Geometry check sheet. Reference: the model listing, model coordinates, mm. A direction names the side the tool comes from. Round coordinates to 2 decimals unless told otherwise and drop trailing zeros. Loops run counter-clockwise (first coordinate to the right, second up) from the corner with the lowest first, then second, coordinate; pieces in that order, holes last. Notation, with made-up numbers: (-10, 75) -> (10, 75) arc R10 ccw to (10, 81) -> close; hole circle Ø6 at (46.25, -24.75). An arc over 180 degrees is marked (long way). Use a Markdown table: item, result. Add a question column.
Q1. Gauge pin test, flat ends, axial feed: P1, Ø7.5, axis at y = -53, z = -84, coming from the +X side; P2, Ø2, axis at y = -48, z = -100.5, coming from the -X side; P3, Ø13, axis at x = 10.5, y = -29, coming from the +Z side. Record the tip position at first contact, or that the pin passes through.
Q2. Sectioned sample at C-C, the plane y = -38. Enter the section's corners in (x, z).
Q3. Sectioned sample at B-B, the plane x = 0. Enter the section's corners in (y, z), then the cut area to 3 significant figures.
Q4. Release check for a two-part mould opening along Z. For faces 6 (the face through (-1, -47, -8)), 7 (the face through (-1, -34, -130)), 8 (the face through (0.1, -26.5, -82)), 9 (the face through (0, -57, -68)) record: released by +Z, released by -Z, zero draft, split by the parting line, or undercut.
Q5. Material ranges on L1, parallel to X at y = -45, z = -81; L2, parallel to Y at x = -32, z = -87; L3, parallel to Z at x = 13, y = -33, recorded low to high.
Q6. Set-up check for faces 1 (the face through (22, -20.25, -70)), 2 (the face through (-0.5, -25.2, -49)), 3 (the face through (0, -30, -24)), 4 (the face through (33, -42, -70)), 5 (the face through (-32, -42, -70)): record each of +Z, -Z, +X, -X, +Y, -Y from which the full face is reachable in a straight line by a thin tool's end or side.
Q7. Sectioned sample at A-A, the plane z = -29.5. Enter the section's corners in (x, y), then the cut area to 3 significant figures.
Q8. Sectioned sample at D-D, the plane y = -49. Enter the section's corners in (x, z).
```python
from build123d import *

# Parameters (mm, degrees)
BOSS_EXTRUDE1_DEPTH     = 8
SKETCH3_R               = 13.75
CUT_EXTRUDE1_DEPTH      = 8
SKETCH4_W               = 80
SKETCH4_H               = 37
BOSS_EXTRUDE2_DEPTH     = 122
SKETCH5_R               = 26.5
CUT_EXTRUDE2_DEPTH      = 16
SKETCH6_R               = 6.5
CUT_EXTRUDE3_DEPTH      = 122
BOSS_EXTRUDE3_START     = 16
BOSS_EXTRUDE3_DEPTH     = 25
BOSS_EXTRUDE4_START     = 108
BOSS_EXTRUDE4_DEPTH     = 14
SKETCH10_W              = 150
SKETCH10_H              = 175
CUT_EXTRUDE4_DEPTH      = 8
CUT_EXTRUDE5_DEPTH      = 141.474196919
CUT_EXTRUDE5_DEPTH_BACK = 141.474196919
SKETCH12_W              = 80
SKETCH12_H              = 0.25
SKETCH13_W              = 15
SKETCH13_H              = 15
CUT_EXTRUDE6_DEPTH      = 122


with BuildPart() as part:
    # Sketch2 → Boss-Extrude1 (new body)
    with BuildSketch(Plane.XY):
        with BuildLine():
            Line((-35, 60), (-35, 50))
            ThreePointArc((-35, 50), (-37.196699141, 44.696699141), (-42.5, 42.5))
            Line((-42.5, 42.5), (-52.5, 42.5))
            ThreePointArc((-52.5, 42.5), (-57.803300859, 40.303300859), (-60, 35))
            Line((-60, 35), (-60, -60))
            ThreePointArc((-60, -60), (-57.803300859, -65.303300859), (-52.5, -67.5))
            Line((-52.5, -67.5), (52.5, -67.5))
            ThreePointArc((52.5, -67.5), (57.803300859, -65.303300859), (60, -60))
            Line((60, -60), (60, 35))
            ThreePointArc((60, 35), (57.803300859, 40.303300859), (52.5, 42.5))
            Line((52.5, 42.5), (42.5, 42.5))
            ThreePointArc((42.5, 42.5), (37.196699141, 44.696699141), (35, 50))
            Line((35, 50), (35, 60))
            ThreePointArc((35, 60), (32.803300859, 65.303300859), (27.5, 67.5))
            Line((27.5, 67.5), (-27.5, 67.5))
            ThreePointArc((-27.5, 67.5), (-32.803300859, 65.303300859), (-35, 60))
        make_face()
    extrude(amount=-BOSS_EXTRUDE1_DEPTH)

    # Sketch3 → Cut-Extrude1 (cut)
    with BuildSketch(Plane.XY):
        with Locations((0, -20)):
            Circle(SKETCH3_R)
    extrude(amount=-CUT_EXTRUDE1_DEPTH, mode=Mode.SUBTRACT)

    # Sketch4 → Boss-Extrude2 (add)
    with BuildSketch(Plane(origin=(0, 0, -8), x_dir=(-1, 0, 0), z_dir=(0, 0, -1))):
        with Locations((0, -38.5)):
            Rectangle(SKETCH4_W, SKETCH4_H)
    extrude(amount=BOSS_EXTRUDE2_DEPTH)

    # Sketch5 → Cut-Extrude2 (cut)
    with BuildSketch(Plane(origin=(0, 0, -8), x_dir=(-1, 0, 0), z_dir=(0, 0, -1))):
        with Locations((0, -20)):
            Circle(SKETCH5_R)
    extrude(amount=CUT_EXTRUDE2_DEPTH, mode=Mode.SUBTRACT)

    # Sketch6 → Cut-Extrude3 (cut)
    with BuildSketch(Plane(origin=(0, 0, -8), x_dir=(-1, 0, 0), z_dir=(0, 0, -1))):
        with Locations((0, -20)):
            Circle(SKETCH6_R)
    extrude(amount=CUT_EXTRUDE3_DEPTH, mode=Mode.SUBTRACT)

    # Sketch8 → Boss-Extrude3 (add)
    with BuildSketch(Plane(origin=(0, 0, -8), x_dir=(-1, 0, 0), z_dir=(0, 0, -1)).offset(BOSS_EXTRUDE3_START)):
        with BuildLine():
            Line((-6.5, -20), (-5, -20))
            ThreePointArc((-5, -20), (0, -25), (5, -20))
            Line((5, -20), (6.5, -20))
            ThreePointArc((6.5, -20), (0, -26.5), (-6.5, -20))
        make_face()
    extrude(amount=BOSS_EXTRUDE3_DEPTH)

    # Sketch9 → Boss-Extrude4 (add)
    with BuildSketch(Plane(origin=(0, 0, -8), x_dir=(-1, 0, 0), z_dir=(0, 0, -1)).offset(BOSS_EXTRUDE4_START)):
        with BuildLine():
            Line((-6.5, -20), (-5, -20))
            ThreePointArc((-5, -20), (0, -25), (5, -20))
            Line((5, -20), (6.5, -20))
            ThreePointArc((6.5, -20), (0, -26.5), (-6.5, -20))
        make_face()
    extrude(amount=BOSS_EXTRUDE4_DEPTH)

    # Sketch10 → Cut-Extrude4 (cut)
    with BuildSketch(Plane.XY):
        Rectangle(SKETCH10_W, SKETCH10_H)
    extrude(amount=-CUT_EXTRUDE4_DEPTH, mode=Mode.SUBTRACT)

    # Sketch12 → Cut-Extrude5 (cut, two sides: drawn at the far end of the back side and taken through both)
    with BuildSketch(Plane.XY.offset(-8).offset(-CUT_EXTRUDE5_DEPTH_BACK)):
        with Locations((0, -20.125)):
            Rectangle(SKETCH12_W, SKETCH12_H)
    extrude(amount=CUT_EXTRUDE5_DEPTH + CUT_EXTRUDE5_DEPTH_BACK, mode=Mode.SUBTRACT)

    # Sketch13 → Cut-Extrude6 (cut)
    with BuildSketch(Plane(origin=(0, 0, -130), x_dir=(-1, 0, 0), z_dir=(0, 0, -1))):
        with Locations((32.5, -49.5)):
            Rectangle(SKETCH13_W, SKETCH13_H)
        with Locations((-32.5, -49.5)):
            Rectangle(SKETCH13_W, SKETCH13_H)
    extrude(amount=-CUT_EXTRUDE6_DEPTH, mode=Mode.SUBTRACT)


solid = part.part
```
Values:
| question | item | result |
|---|---|---|
| 1 | P1 | x = 25 |
| 1 | P2 | x = -25 |
| 1 | P3 | z = -24 |
| 2 | outline | (-40, -130) -> (40, -130) -> (40, -8) -> (19.45, -8) -> (19.45, -24) -> (-19.45, -24) -> (-19.45, -8) -> (-40, -8) -> close |
| 3 | outline | (-57, -130) -> (-25, -130) -> (-25, -116) -> (-26.5, -116) -> (-26.5, -49) -> (-25, -49) -> (-25, -24) -> (-46.5, -24) -> (-46.5, -8) -> (-57, -8) -> close |
| 3 | area | 3,460 mm^2 |
| 4 | face 6 | released by +Z |
| 4 | face 7 | released by -Z |
| 4 | face 8 | undercut |
| 4 | face 9 | zero draft |
| 5 | L1 | -25 to 25 |
| 5 | L2 | -42 to -20.25 |
| 5 | L3 | -130 to -24 |
| 6 | face 1 | +Z, -Z, +X, -X, +Y |
| 6 | face 2 | +Y |
| 6 | face 3 | +Z, +Y |
| 6 | face 4 | +Z, -Z, +X, -Y |
| 6 | face 5 | +Z, -Z, -X, -Y |
| 7 | outline | (-40, -42) -> (-25, -42) -> (-25, -57) -> (25, -57) -> (25, -42) -> (40, -42) -> (40, -20.25) -> (4.99, -20.25) arc R5 cw to (-4.99, -20.25) -> (-40, -20.25) -> close |
| 7 | area | 2,450 mm^2 |
| 8 | outline | (-25, -130) -> (25, -130) -> (25, -8) -> (-25, -8) -> close |
